from build123d import *

# Parameters (mm, degrees)
SKETCH_1_W          = 10
SKETCH_1_H          = 50
EXTRUDE_1_DEPTH     = 2
SKETCH_2_W          = 50
SKETCH_2_H          = 2
EXTRUDE_2_DEPTH     = 3
SKETCH_3_W          = 3
SKETCH_3_H          = 50
EXTRUDE_3_DEPTH     = 52
SKETCH_4_W          = 50
SKETCH_4_H          = 2
EXTRUDE_4_DEPTH     = 10
SKETCH_5_R          = 2
CUT_EXTRUDE_1_DEPTH = 61.041652209
SKETCH_6_W          = 50
SKETCH_6_H          = 54
EXTRUDE_5_DEPTH     = 1.5
SKETCH_7_W          = 50
SKETCH_7_H          = 50
CUT_EXTRUDE_2_DEPTH = 1.5
SKETCH_8_W          = 50
SKETCH_8_H          = 2
CUT_EXTRUDE_3_DEPTH = 1.5


with BuildPart() as part:
    # 草图1 → 凸台-拉伸1 (new body)
    with BuildSketch(Plane(origin=(0, 0, 0), x_dir=(1, 0, 0), z_dir=(0, 1, 0))):
        Rectangle(SKETCH_1_W, SKETCH_1_H)
    extrude(amount=EXTRUDE_1_DEPTH)

    # 草图2 → 凸台-拉伸2 (add)
    with BuildSketch(Plane(origin=(5, 0, 0), x_dir=(0, 0, -1), z_dir=(1, 0, 0))):
        with Locations((0, 1)):
            Rectangle(SKETCH_2_W, SKETCH_2_H)
    extrude(amount=EXTRUDE_2_DEPTH)

    # 草图3 → 凸台-拉伸3 (add)
    with BuildSketch(Plane.XZ):
        with Locations((6.5, 0)):
            Rectangle(SKETCH_3_W, SKETCH_3_H)
    extrude(amount=EXTRUDE_3_DEPTH)

    # 草图4 → 凸台-拉伸4 (add)
    with BuildSketch(Plane.ZY.offset(-5)):
        with Locations((0, -51)):
            Rectangle(SKETCH_4_W, SKETCH_4_H)
    extrude(amount=EXTRUDE_4_DEPTH)

    # 草图5 → 切除-拉伸1 (cut, through all)
    with BuildSketch(Plane(origin=(0, -52, 0), x_dir=(-1, 0, 0), z_dir=(0, -1, 0))):
        with Locations(Location((-1.5, -15, 0), (0, 0, 90))):
            Circle(SKETCH_5_R)
        with Locations(Location((-1.5, -5, 0), (0, 0, 90))):
            Circle(SKETCH_5_R)
        with Locations(Location((-1.5, 5, 0), (0, 0, 90))):
            Circle(SKETCH_5_R)
        with Locations(Location((-1.5, 15, 0), (0, 0, 90))):
            Circle(SKETCH_5_R)
    extrude(amount=-CUT_EXTRUDE_1_DEPTH, mode=Mode.SUBTRACT)

    # 草图6 → 凸台-拉伸5 (add)
    with BuildSketch(Plane(origin=(8, 0, 0), x_dir=(0, 0, -1), z_dir=(1, 0, 0))):
        with Locations((0, -25)):
            Rectangle(SKETCH_6_W, SKETCH_6_H)
    extrude(amount=EXTRUDE_5_DEPTH)

    # 草图7 → 切除-拉伸2 (cut)
    with BuildSketch(Plane.ZY.offset(-5)):
        with Locations((0, -25)):
            Rectangle(SKETCH_7_W, SKETCH_7_H)
    extrude(amount=-CUT_EXTRUDE_2_DEPTH, mode=Mode.SUBTRACT)

    # 草图8 → 切除-拉伸3 (cut)
    with BuildSketch(Plane.ZY.offset(5)):
        with Locations((0, -51)):
            Rectangle(SKETCH_8_W, SKETCH_8_H)
        with Locations((0, 1)):
            Rectangle(SKETCH_8_W, SKETCH_8_H)
    extrude(amount=-CUT_EXTRUDE_3_DEPTH, mode=Mode.SUBTRACT)


solid = part.part
For this review, take the finished solid that the model builds, in its own axes (mm). A direction names the side the tool comes from. Coordinates: 2 decimals unless noted, no trailing zeros. Order: outer loops, then holes, each group sorted by start corner. A loop starts at its lowest first (then second) coordinate and runs counter-clockwise, first axis right, second up. Notation, with made-up numbers: (-1.5, -13.5) - (4.5, -13.5) arc R25 cw to (4.5, 0.5) - close; hole circle Ø10 at (-5, 70.25). An arc over 180 degrees is marked (long way). Use one line per item in the form item = value.
Q1. For faces 1 (the cylindrical face through (0.3, 1, 6.6)), 2 (the flat face through (6.5, -25, 0)), list the 3-axis set-ups (+Z, -Z, +X, -X, +Y, -Y) from which the entire face can be reached by the end or side of a thin tool; tool diameter is ignored.
Checked values:
face_1 = +Y, -Y
face_2 = +Z, -Z, -X
Q2. For P1, Ø3, axis at y = -24, z = 0, coming from the -X side, flat-tipped, find the tip position at first contact; note if it passes through.
Checked values:
P1 = 6.5
Q3. Draft analysis for pull direction Z (two halves, no side actions). For faces 3 (the cylindrical face through (0.3, -51, -13.4)), 4 (the cylindrical face through (0.3, 1, 16.6)), 5 (the flat face through (7, -25, -25)), 6 (the flat face through (3, -52, 0)), state which applies: +Z half, -Z half, draft (parallel to the pull), parting line (faces both ways), or undercut.
Checked values:
face_3 = undercut
face_4 = undercut
face_5 = -Z half
face_6 = draft
Q4. Consider section A-A (z = 5). Give the boundary of the cut face in (x, y), then the cut area to 3 significant figures.
Checked values:
outline = (-3.5, -52) - (-0.5, -52) - (-0.5, -50) - (-3.5, -50) - close; (-3.5, 0) - (-0.5, 0) - (-0.5, 2) - (-3.5, 2) - close; (3.5, -52) - (9.5, -52) - (9.5, 2) - (3.5, 2) - (3.5, 0) - (6.5, 0) - (6.5, -50) - (3.5, -50) - close
area = 186 mm2
Q5. For probe 1 along Y at (x, z) = (6, -21); probe 2 along X at (y, z) = (-50.35, 5); probe 3 along X at (y, z) = (-37, 19), list the stretches that pass through material, from the lowest coordinate up. Write a range as from..to.
Checked values:
probe_1 = -52..-50, 0..2
probe_2 = -3.5..-0.5, 3.5..9.5
probe_3 = 6.5..9.5
Q6. Consider section C-C (y = -7). Give the boundary of the cut face in (x, z).
Checked values:
outline = (6.5, -25) - (9.5, -25) - (9.5, 25) - (6.5, 25) - close
Q7. Consider section B-B (x = 1.5). Give the number of separate pieces and of enclosed holes in the cut face, then the cut area to 3 significant figures.
Checked values:
separate_pieces = 10
enclosed_holes = 0
area = 136 mm2
